Build history of the part. All positions in model axes, mm. Round coordinates to 2 decimals unless told otherwise and drop trailing zeros. One line per question, with ' | ' between items. Start each with the question number.
from build123d import *

# Parameters (mm, degrees)
BOSS_EXTRUDE1_DEPTH = 304.8
MIRROR3_START       = -304.8
MIRROR3_DEPTH       = 609.6


# Read off the part's stored shape, not the designer's step: Mirror3
with BuildPart() as part:
    # Sketch3 → Boss-Extrude1 (new, symmetric)
    with BuildSketch(Plane.XY):
        with BuildLine():
            Line((0, 8), (0, 3.5))
            ThreePointArc((0, 3.5), (-2.474873734, 2.474873734), (-3.5, 0))
            Line((-3.5, 0), (-8, 0))
            Line((-8, 0), (-8, 4.600266817))
            ThreePointArc((-8, 4.600266817), (-8.096672994, 5.086274776), (-8.371974388, 5.498292429))
            Line((-8.371974388, 5.498292429), (-13.873681959, 11))
            Line((-13.873681959, 11), (-17.7902, 11))
            Line((-17.7902, 11), (-17.7902, 6.2098))
            Line((-17.7902, 6.2098), (-17.0282, 6.2098))
            Line((-17.0282, 6.2098), (-17.0282, 4.508))
            ThreePointArc((-17.0282, 4.508), (-17.176989755, 4.148789755), (-17.5362, 4))
            Line((-17.5362, 4), (-18.8951, 4))
            ThreePointArc((-18.8951, 4), (-19.676382283, 4.323617717), (-20, 5.1049))
            Line((-20, 5.1049), (-20, 16.68))
            ThreePointArc((-20, 16.68), (-19.027594514, 19.027594514), (-16.68, 20))
            Line((-16.68, 20), (-5.1049, 20))
            ThreePointArc((-5.1049, 20), (-4.323617717, 19.676382283), (-4, 18.8951))
            Line((-4, 18.8951), (-4, 17.5362))
            ThreePointArc((-4, 17.5362), (-4.148789755, 17.176989755), (-4.508, 17.0282))
            Line((-4.508, 17.0282), (-6.2098, 17.0282))
            Line((-6.2098, 17.0282), (-6.2098, 17.7902))
            Line((-6.2098, 17.7902), (-11, 17.7902))
            Line((-11, 17.7902), (-11, 13.873681959))
            Line((-11, 13.873681959), (-5.498292429, 8.371974388))
            ThreePointArc((-5.498292429, 8.371974388), (-5.086274776, 8.096672994), (-4.600266817, 8))
            Line((-4.600266817, 8), (0, 8))
        make_face()
        with BuildLine():
            Line((-12.065, 18.73), (-12.065, 12.065))
            Line((-12.065, 12.065), (-18.73, 12.065))
            Line((-18.73, 12.065), (-18.73, 16.19))
            ThreePointArc((-18.73, 16.19), (-17.986051224, 17.986051224), (-16.19, 18.73))
            Line((-16.19, 18.73), (-12.065, 18.73))
        make_face(mode=Mode.SUBTRACT)
    extrude(amount=BOSS_EXTRUDE1_DEPTH, both=True)

    # Mirror1: part across plane


with BuildPart() as part_1:
    add(part.part)
    add(part.part.mirror(Plane(origin=(0, 0, 304.8), x_dir=(0, 0, 1), z_dir=(1, 0, 0))))

    # Mirror3 outline → Mirror3 (add)
    with BuildSketch(Plane.XY.offset(MIRROR3_START)):
        with BuildLine():
            Line((-8, 0), (-8, -4.600266817))
            ThreePointArc((-8, -4.600266817), (-8.096672994, -5.086274776), (-8.371974388, -5.498292429))
            Line((-8.371974388, -5.498292429), (-13.873681959, -11))
            Line((-13.873681959, -11), (-17.7902, -11))
            Line((-17.7902, -11), (-17.7902, -6.2098))
            Line((-17.7902, -6.2098), (-17.0282, -6.2098))
            Line((-17.0282, -6.2098), (-17.0282, -4.508))
            ThreePointArc((-17.0282, -4.508), (-17.176989755, -4.148789755), (-17.5362, -4))
            Line((-17.5362, -4), (-18.8951, -4))
            ThreePointArc((-18.8951, -4), (-19.676382283, -4.323617717), (-20, -5.1049))
            Line((-20, -5.1049), (-20, -16.68))
            ThreePointArc((-20, -16.68), (-19.027594514, -19.027594514), (-16.68, -20))
            Line((-16.68, -20), (-5.1049, -20))
            ThreePointArc((-5.1049, -20), (-4.323617717, -19.676382283), (-4, -18.8951))
            Line((-4, -18.8951), (-4, -17.5362))
            ThreePointArc((-4, -17.5362), (-4.148789755, -17.176989755), (-4.508, -17.0282))
            Line((-4.508, -17.0282), (-6.2098, -17.0282))
            Line((-6.2098, -17.0282), (-6.2098, -17.7902))
            Line((-6.2098, -17.7902), (-11, -17.7902))
            Line((-11, -17.7902), (-11, -13.873681959))
            Line((-11, -13.873681959), (-5.498292429, -8.371974388))
            ThreePointArc((-5.498292429, -8.371974388), (-5.086274776, -8.096672994), (-4.600266817, -8))
            Line((-4.600266817, -8), (4.600266817, -8))
            ThreePointArc((4.600266817, -8), (5.086274776, -8.096672994), (5.498292429, -8.371974388))
            Line((5.498292429, -8.371974388), (11, -13.873681959))
            Line((11, -13.873681959), (11, -17.7902))
            Line((11, -17.7902), (6.2098, -17.7902))
            Line((6.2098, -17.7902), (6.2098, -17.0282))
            Line((6.2098, -17.0282), (4.508, -17.0282))
            ThreePointArc((4.508, -17.0282), (4.148789755, -17.176989755), (4, -17.5362))
            Line((4, -17.5362), (4, -18.8951))
            ThreePointArc((4, -18.8951), (4.323617717, -19.676382283), (5.1049, -20))
            Line((5.1049, -20), (16.68, -20))
            ThreePointArc((16.68, -20), (19.027594514, -19.027594514), (20, -16.68))
            Line((20, -16.68), (20, -5.1049))
            ThreePointArc((20, -5.1049), (19.676382283, -4.323617717), (18.8951, -4))
            Line((18.8951, -4), (17.5362, -4))
            ThreePointArc((17.5362, -4), (17.176989755, -4.148789755), (17.0282, -4.508))
            Line((17.0282, -4.508), (17.0282, -6.2098))
            Line((17.0282, -6.2098), (17.7902, -6.2098))
            Line((17.7902, -6.2098), (17.7902, -11))
            Line((17.7902, -11), (13.873681959, -11))
            Line((13.873681959, -11), (8.371974388, -5.498292429))
            ThreePointArc((8.371974388, -5.498292429), (8.096672994, -5.086274776), (8, -4.600266817))
            Line((8, -4.600266817), (8, 0))
            Line((8, 0), (3.5, 0))
            ThreePointArc((3.5, 0), (0, -3.5), (-3.5, 0))
            Line((-3.5, 0), (-8, 0))
        make_face()
        with BuildLine():
            Line((-12.065, -12.065), (-12.065, -18.73))
            Line((-12.065, -18.73), (-16.19, -18.73))
            ThreePointArc((-16.19, -18.73), (-17.986051224, -17.986051224), (-18.73, -16.19))
            Line((-18.73, -16.19), (-18.73, -12.065))
            Line((-18.73, -12.065), (-12.065, -12.065))
        make_face(mode=Mode.SUBTRACT)
        with BuildLine():
            Line((12.065, -18.73), (12.065, -12.065))
            Line((12.065, -12.065), (18.73, -12.065))
            Line((18.73, -12.065), (18.73, -16.19))
            ThreePointArc((18.73, -16.19), (17.986051224, -17.986051224), (16.19, -18.73))
            Line((16.19, -18.73), (12.065, -18.73))
        make_face(mode=Mode.SUBTRACT)
    extrude(amount=MIRROR3_DEPTH)


solid = part_1.part
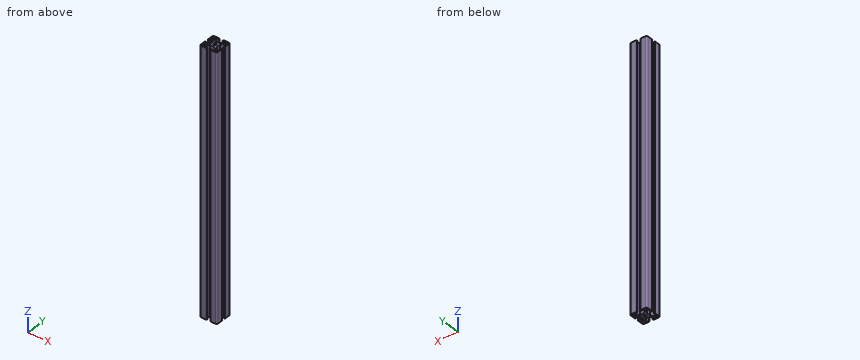
Item 1: Wall check: line 1 along X through (y, z) = (-5, 100) (3 decimals); line 2 along X through (y, z) = (14.5, 21) (3 decimals); line 3 along Y through (x, z) = (-5.5, -142). Give the ranges that are in metal, low to high. Write a range as [from, to].
Item 2: Cut at A-A on z = -62. Count the separate pieces of the cut face and the enclosed holes in it, then the cut area to 3 significant figures.
Item 3: Flat gauge pin, fed straight in: pin 1 (0.6 mm diameter, centred on x = 17.5, z = -24.5, fed in from +Y). Where does the tip first touch, or does it go through?
Results found:
1) line 1: x = [-19.995, -17.028], [-8.065, 8.065], [17.028, 19.995] | line 2: x = [-20, -18.73], [-12.065, -11], [11, 12.065], [18.73, 20] | line 3: y = [-20, -17.03], [-8.37, 8.37], [17.03, 20]
2) separate pieces: 1 | enclosed holes: 5 | area: 597 mm^2
3) pin 1: stops at y = 19.96
